The figure shows three views and two pictorial views of one solid part (mm, origin at its lowest corner). Answer the questions. A direction names the side the tool comes from. Give positions to 0.01 mm unless a question says otherwise; leave off trailing zeros. Order: outer loops, then holes, each group sorted by start corner. A loop starts at its lowest first (then second) coordinate and runs counter-clockwise, first axis right, second up. Notation, with made-up numbers: (87, 63) - (99, 63) arc R16 ccw to (99, 76) - close; hole circle Ø7 at (-26, -9). An arc over 180 degrees is marked (long way). Answer as a JSON object with one key per item and string values. Group by question number.
Q1. Given pin 1 (4.5 mm diameter, centred on x = 37.5, y = 16, fed in from +Z); pin 2 (7 mm diameter, centred on x = 88, z = 21.5, fed in from +Y); pin 3 (4.5 mm diameter, centred on x = 57.5, y = 16, fed in from -Z), each flat-ended and moving along its own axis, determine where each tip first touches the part or whether it passes through.
Q2. For the marked faces 1, 2, 3 and 4, determine the directions among +Z, -Z, +X, -X, +Y, -Y from which every point of the face is accessible in a straight line to the end or side of a thin tool.
Q3. A cutting plane is placed at B-B, the plane x = 37.5. Give the vertices of the cut face in (y, z), and give its area (3 significant figures).
Q4. A cutting plane is placed at C-C, the plane y = 16. Give the vertices of the cut face in (x, z).
Q5. A cutting plane is placed at A-A, the plane z = 22.5. Give the vertices of the cut face in (x, y).
Q6. A cutting plane is placed at D-D, the plane x = 6.5. Give the vertices of the cut face in (y, z), and give its area (3 significant figures).
Q7. Consider line 1 (Y direction, x = 57.5, z = 29); line 2 (X direction, y = 16, z = 27); line 3 (X direction, y = 0.75, z = 22.5). Determine where each line is inside the solid, lowest interval first.
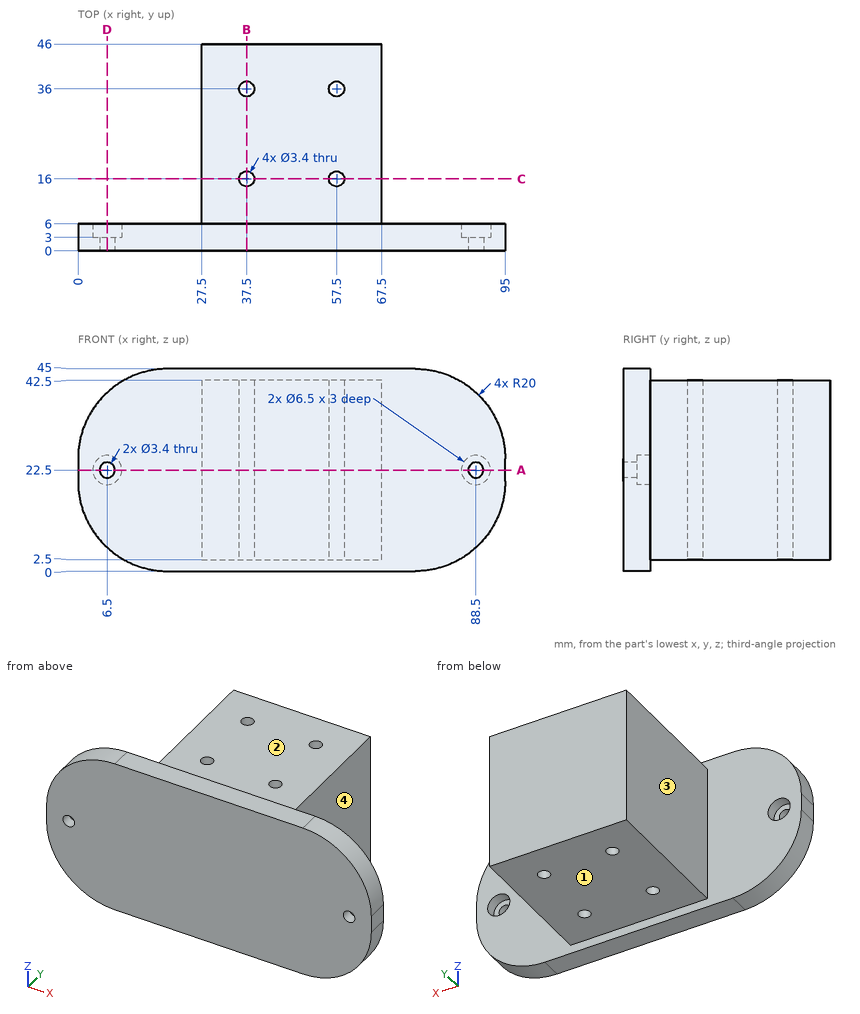
Reply:
{
 "1": {"pin 1": "stops at z = 42.5", "pin 2": "stops at y = 6", "pin 3": "stops at z = 2.5"},
 "2": {"face 1": "-Z, +X, -X, +Y", "face 2": "+Z, +X, -X, +Y", "face 3": "+Z, -Z, -X, +Y", "face 4": "+Z, -Z, +X, +Y"},
 "3": {"outline": "(0, 0) - (6, 0) - (6, 2.5) - (14.3, 2.5) - (14.3, 42.5) - (6, 42.5) - (6, 45) - (0, 45) - close; (17.7, 2.5) - (34.3, 2.5) - (34.3, 42.5) - (17.7, 42.5) - close; (37.7, 2.5) - (46, 2.5) - (46, 42.5) - (37.7, 42.5) - close", "area": "1,600 mm^2"},
 "4": {"outline": "(27.5, 2.5) - (35.8, 2.5) - (35.8, 42.5) - (27.5, 42.5) - close; (39.2, 2.5) - (55.8, 2.5) - (55.8, 42.5) - (39.2, 42.5) - close; (59.2, 2.5) - (67.5, 2.5) - (67.5, 42.5) - (59.2, 42.5) - close"},
 "5": {"outline": "(0, 0) - (4.8, 0) - (4.8, 3) - (3.25, 3) - (3.25, 6) - (0, 6) - close; (8.2, 0) - (86.8, 0) - (86.8, 3) - (85.25, 3) - (85.25, 6) - (67.5, 6) - (67.5, 46) - (27.5, 46) - (27.5, 6) - (9.75, 6) - (9.75, 3) - (8.2, 3) - close; (90.2, 0) - (95, 0) - (95, 6) - (91.75, 6) - (91.75, 3) - (90.2, 3) - close; hole circle Ø3.4 at (37.5, 16); hole circle Ø3.4 at (37.5, 36); hole circle Ø3.4 at (57.5, 16); hole circle Ø3.4 at (57.5, 36)"},
 "6": {"outline": "(0, 5.24) - (6, 5.24) - (6, 19.25) - (3, 19.25) - (3, 20.8) - (0, 20.8) - close; (0, 24.2) - (3, 24.2) - (3, 25.75) - (6, 25.75) - (6, 39.76) - (0, 39.76) - close", "area": "177 mm^2"},
 "7": {"line 1": "y = 0 to 14.3, 17.7 to 34.3, 37.7 to 46", "line 2": "x = 27.5 to 35.8, 39.2 to 55.8, 59.2 to 67.5", "line 3": "x = 0 to 4.8, 8.2 to 86.8, 90.2 to 95"}
}
